Geometry: final body of the model. Coordinates: model frame, mm. A direction names the side the tool comes from. Give positions to 0.01 mm unless a question says otherwise; leave off trailing zeros. Loops run counter-clockwise (first coordinate to the right, second up) from the corner with the lowest first, then second, coordinate; pieces in that order, holes last. Notation, with made-up numbers: (-3.75, 4.5) -> (1.25, 4.5) arc R28 ccw to (1.25, 35.5) -> close; hole circle Ø9 at (-16.5, 51.5). An arc over 180 degrees is marked (long way). Answer in a Markdown table with one row per item. Add a question column.
1) Draft query along Z for faces 1 (the flat face through (-350, -47, 887)), 2 (the cylindrical face through (-299.67, 98.31, 1.5)), 3 (the flat face through (-5, 2, 1800)), 4 (the cylindrical face through (230.887, -142.605, 869.404)). Return one class per face: +Z half, -Z half, draft (parallel to the pull), parting line (faces both ways), or undercut.
2) Section query A-A (z = 1650). Return the cut outline in (x, y), plus the area to 3 significant figures.
3) Section query C-C (y = -31.5). Return the cut outline in (x, z), plus the area to 3 significant figures.
4) Section query B-B (x = 0). Return the cut outline in (y, z).
5) Line query: line 1 (Z direction, x = -240, y = -141); line 2 (Z direction, x = 295, y = -81.5); line 3 (Y direction, x = 117, z = 1161.5). Output: solid intervals per line, ascending. Write a range as from..to.
6) Access query for faces 5 (the cylindrical face through (-27.098, -142.605, 327.972)), 6 (the flat face through (290.032, 88.755, 904.855)), 7 (the flat face through (3, 150, 887)). Directions: +Z, -Z, +X, -X, +Y, -Y. A direction counts if a zero-diameter tool reaches every point of the face in a straight line with its end or side. Return the directions, or none.
7) First-contact query: P1, Ø5, axis at y = 90, z = 859.5, coming from the +X side; P2, Ø12, axis at y = 104.5, z = 362.5, coming from the -X side; P3, Ø1.5, axis at x = -175, y = -84, coming from the -Z side. Flat tips, straight axial feed; report the tip coordinate or a pass-through.
8) Section query D-D (z = 1402.5). Return the cut outline in (x, y).
```python
from build123d import *

# Parameters (mm, degrees)
F1_DEPTH  = 1800
F2_R      = 5
F3_W      = 90
F3_H      = 130
F4_DEPTH  = 25
F6_DEPTH  = 1790
F7_R      = 37.5
F7_R_2    = 65
F7_R_3    = 70
F8_DEPTH  = 15
F10_START = 1775
F10_DEPTH = 25


with BuildPart() as f1:
    # F0 (on Top) → F1 (new body)
    with BuildSketch(Plane.XY):
        Polygon((-350, -150), (350, -150), (350, 50), (250, 150), (0, 150), (-250, 150), (-350, 50), align=None)
    extrude(amount=F1_DEPTH)

    # F2
    f2_edges = [f1.edges().sort_by_distance(p)[0] for p in [
        (-350, -150, 900),
        (0, -150, 1800),
        (350, -150, 900),
        (0, -150, 0),
        (350, -50, 0),
        (-350, -50, 0),
        (-300, 100, 0),
        (0, 150, 0),
        (300, 100, 0),
        (350, 50, 900),
        (250, 150, 900),
        (300, 100, 1800),
        (0, 150, 1800),
        (350, -50, 1800),
        (-300, 100, 1800),
        (-350, -50, 1800),
        (-350, 50, 900),
        (-250, 150, 900),
    ]]
    fillet(f2_edges, radius=F2_R)

    # F3 (on face) → F4 (cut)
    with BuildSketch(Plane.XZ.offset(150)):
        with Locations((-45, 1280)):
            Rectangle(F3_W, F3_H)
        with Locations((45, 1280)):
            Rectangle(F3_W, F3_H)
    extrude(amount=-F4_DEPTH, mode=Mode.SUBTRACT)

    # F5 (on face) → F6 (cut)
    with BuildSketch(Plane.XY.offset(1800)):
        Polygon((335, 43.7867965644), (243.7867965644, 135), (-243.7867965644, 135), (-335, 43.7867965644), (-335, -135), (335, -135), align=None)
    extrude(amount=-F6_DEPTH, mode=Mode.SUBTRACT)

    # F7 (on face) → F8 (cut, through all)
    with BuildSketch(Plane.XZ.offset(150)):
        with Locations((240, 1650)):
            Circle(F7_R)
        with Locations((240, 1100)):
            Circle(F7_R_2)
        with BuildLine():
            ThreePointArc((125, 450), (88.3883476483, 538.3883476483), (0, 575))
            Line((0, 575), (0, 325))
            ThreePointArc((0, 325), (88.3883476483, 361.6116523517), (125, 450))
        make_face()
        with BuildLine():
            Line((0, 325), (0, 575))
            ThreePointArc((0, 575), (-125, 450), (0, 325))
        make_face()
        with Locations((240, 800)):
            Circle(F7_R_3)
        with Locations((-240, 1650)):
            Circle(F7_R)
        with Locations((-240, 1100)):
            Circle(F7_R_2)
        with Locations((-240, 800)):
            Circle(F7_R_3)
    extrude(amount=-F8_DEPTH, mode=Mode.SUBTRACT)

    # F9 (on Top) → F10 (join)
    with BuildSketch(Plane.XY.offset(F10_START)):
        Polygon((340, 45.8578643763), (245.8578643763, 140), (-245.8578643763, 140), (-340, 45.8578643763), (-340, -140), (340, -140), align=None)
    extrude(amount=F10_DEPTH)


solid = f1.part
```
Evaluation:
| question | item | result |
|---|---|---|
| 1 | face 1 | draft |
| 1 | face 2 | -Z half |
| 1 | face 3 | +Z half |
| 1 | face 4 | undercut |
| 2 | outline | (-350, -145) arc R5 ccw to (-345, -150) -> (-277.5, -150) -> (-277.5, -135) -> (-335, -135) -> (-335, 43.79) -> (-243.79, 135) -> (243.79, 135) -> (335, 43.79) -> (335, -135) -> (277.5, -135) -> (277.5, -150) -> (345, -150) arc R5 ccw to (350, -145) -> (350, 47.93) arc R5 ccw to (348.54, 51.46) -> (251.46, 148.54) arc R5 ccw to (247.93, 150) -> (-247.93, 150) arc R5 ccw to (-251.46, 148.54) -> (-348.54, 51.46) arc R5 ccw to (-350, 47.93) -> close; (-202.5, -150) -> (202.5, -150) -> (202.5, -135) -> (-202.5, -135) -> close |
| 2 | area | 25,200 mm² |
| 3 | outline | (-350, 5) arc R5 ccw to (-345, 0) -> (345, 0) arc R5 ccw to (350, 5) -> (350, 1795) arc R5 ccw to (345, 1800) -> (-345, 1800) arc R5 ccw to (-350, 1795) -> close; hole (-335, 10) -> (335, 10) -> (335, 1775) -> (-335, 1775) -> close |
| 3 | area | 77,400 mm² |
| 4 | outline | (-150, 5) arc R5 ccw to (-145, 0) -> (145, 0) arc R5 ccw to (150, 5) -> (150, 1795) arc R5 ccw to (145, 1800) -> (-145, 1800) arc R5 ccw to (-150, 1795) -> (-150, 1345) -> (-135, 1345) -> (-135, 1775) -> (135, 1775) -> (135, 10) -> (-135, 10) -> (-135, 325) -> (-150, 325) -> close; (-150, 575) -> (-135, 575) -> (-135, 1215) -> (-150, 1215) -> close |
| 5 | line 1 | 0..730, 870..1035, 1165..1612.5, 1687.5..1800 |
| 5 | line 2 | 0..10, 1775..1800 |
| 5 | line 3 | -150..-135, 135..150 |
| 6 | face 5 | -Y |
| 6 | face 6 | none |
| 6 | face 7 | +Z, -Z, +X, -X, +Y |
| 7 | P1 | x = 312.5 |
| 7 | P2 | x = -301.5 |
| 7 | P3 | z = 0 |
| 8 | outline | (-350, -145) arc R5 ccw to (-345, -150) -> (345, -150) arc R5 ccw to (350, -145) -> (350, 47.93) arc R5 ccw to (348.54, 51.46) -> (251.46, 148.54) arc R5 ccw to (247.93, 150) -> (-247.93, 150) arc R5 ccw to (-251.46, 148.54) -> (-348.54, 51.46) arc R5 ccw to (-350, 47.93) -> close; hole (-335, -135) -> (335, -135) -> (335, 43.79) -> (243.79, 135) -> (-243.79, 135) -> (-335, 43.79) -> close |
